Design review of the part shown in the three views and the two pictorial views. Dimensions are in mm from the part's minimum x, y and z. A direction names the side the tool comes from. Give positions to 0.01 mm unless a question says otherwise; leave off trailing zeros. Loops run counter-clockwise (first coordinate to the right, second up) from the corner with the lowest first, then second, coordinate; pieces in that order, holes last. Notation, with made-up numbers: (7.25, 89) - (19.25, 89) arc R17 cw to (19.25, 121) - close; hole circle Ø4 at (51, -20). An arc over 180 degrees is marked (long way). Answer in a Markdown table with one row per item.
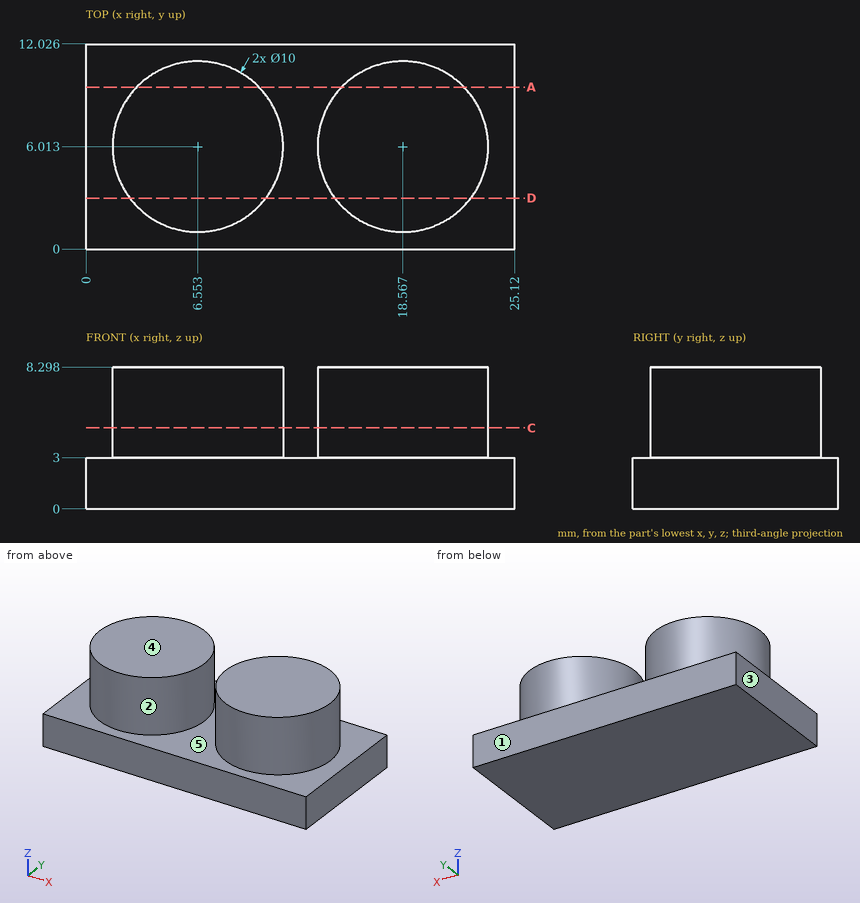
1. Clearance check with flat-ended pins moving along their axes: pin 1 (2 mm diameter, centred on y = 2, z = 5.5, fed in from -X); pin 2 (2 mm diameter, centred on y = 3.5, z = 6.5, fed in from -X); pin 3 (1.5 mm diameter, centred on x = 7.5, z = 4.5, fed in from +Y). State where each tip first meets the part, or that it passes through.
Values:
| item | result |
|---|---|
| pin 1 | stops at x = 2.56 |
| pin 2 | stops at x = 1.79 |
| pin 3 | stops at y = 11.01 |
2. We need section A-A, the plane y = 9.5. Give the boundary of the cut face in (x, z).
Values:
| item | result |
|---|---|
| outline | (0, 0) - (25.12, 0) - (25.12, 3) - (22.15, 3) - (22.15, 8.3) - (14.98, 8.3) - (14.98, 3) - (10.14, 3) - (10.14, 8.3) - (2.97, 8.3) - (2.97, 3) - (0, 3) - close |
3. Mouldability with a two-part tool opening along X and no side actions: class the marked faces 3, 4 and 5 as released by +X, released by -X, zero draft, split by the parting line, or undercut.
Values:
| item | result |
|---|---|
| face 3 | released by -X |
| face 4 | zero draft |
| face 5 | undercut |
4. For the marked faces 1 and 2, list the 3-axis set-ups (+Z, -Z, +X, -X, +Y, -Y) from which the entire face can be reached by the end or side of a thin tool; tool diameter is ignored.
Values:
| item | result |
|---|---|
| face 1 | +Z, -Z, +X, -X, +Y |
| face 2 | +Z |
5. We need section C-C, the plane z = 4.75. Give the boundary of the cut face in (x, y).
Values:
| item | result |
|---|---|
| outline | circle Ø10 at (6.55, 6.01); circle Ø10 at (18.57, 6.01) |
6. Wall thickness on line 1 (Z direction, x = 1.75, y = 11); line 2 (X direction, y = 9, z = 3.25) (1 decimal); line 3 (X direction, y = 6.75, z = 6.5): over which ranges is each line inside the solid? List them lowest first. Write a range as [from, to].
Values:
| item | result |
|---|---|
| line 1 | z = [0, 3] |
| line 2 | x = [2.5, 10.6], [14.6, 22.6] |
| line 3 | x = [1.61, 11.5], [13.62, 23.51] |
7. We need section D-D, the plane y = 3. Give the boundary of the cut face in (x, z), and give its area (3 significant figures).
Values:
| item | result |
|---|---|
| outline | (0, 0) - (25.12, 0) - (25.12, 3) - (22.56, 3) - (22.56, 8.3) - (14.58, 8.3) - (14.58, 3) - (10.54, 3) - (10.54, 8.3) - (2.56, 8.3) - (2.56, 3) - (0, 3) - close |
| area | 160 mm^2 |
